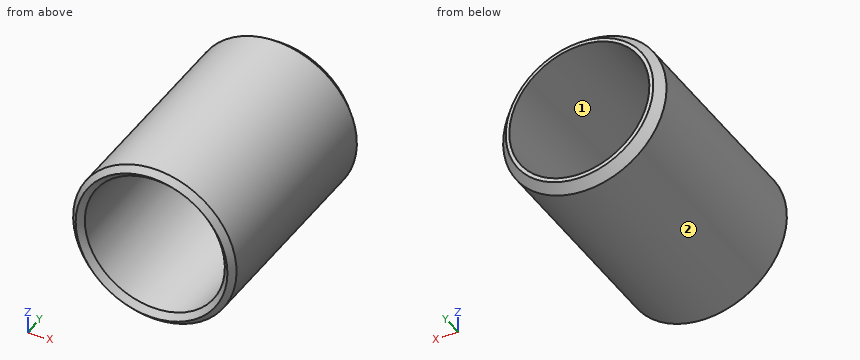
```python
from build123d import *

# Parameters (mm, degrees)
CROQUIS2_R            = 6
CORTAR_EXTRUIR1_DEPTH = 60
CHAFL_N2_SIZE         = 0.5
CHAFL_N2_SIZE_2       = 0.354903907


with BuildPart() as part:
    # Croquis1 → Revolución1 (revolve)
    with BuildSketch(Plane.XY, mode=Mode.PRIVATE) as revoluci_n1_sk:
        Polygon((-7, 18.808246407), (-7, 0), (0, 0), (0, 20), (-6, 20), align=None)
    revolve(revoluci_n1_sk.sketch.rotate(Axis((0, 0, 0), (0, 1, 0)), 270), axis=Axis((0, 0, 0), (0, 1, 0)))

    # Croquis2 → Cortar-Extruir1 (cut)
    with BuildSketch(Plane(origin=(0, 20, 0), x_dir=(1, 0, 0), z_dir=(0, 1, 0))):
        with Locations(Location((0, 0, 0), (0, 0, 270))):
            Circle(CROQUIS2_R)
    extrude(amount=-CORTAR_EXTRUIR1_DEPTH, mode=Mode.SUBTRACT)

    # Chaflán2
    # the kernel refuses this chamfer: 0.5, 0.354903907 mm, written as the material it takes off along each edge
    with BuildSketch(Plane(origin=(0, 0, 0), x_dir=(0, 0, 1), z_dir=(-1, 0, 0))) as chafl_n2_piece_1:
        Polygon((6 + CHAFL_N2_SIZE, 0), (6, CHAFL_N2_SIZE), (6, 0), align=None)
    revolve(axis=Axis((0, 0, 0), (0, 1, 0)), mode=Mode.SUBTRACT)
    with BuildSketch(Plane(origin=(0, 0, 0), x_dir=(0, 0, -1), z_dir=(1, 0, 0))) as chafl_n2_piece_2:
        Polygon((7, CHAFL_N2_SIZE), (7 - CHAFL_N2_SIZE, 0), (7, 0), align=None)
    revolve(axis=Axis((0, 0, 0), (0, 1, 0)), mode=Mode.SUBTRACT)
    with BuildSketch(Plane(origin=(0, 20, 0), x_dir=(0, 0, 1), z_dir=(-1, 0, 0))) as chafl_n2_piece_3:
        Polygon((6 + CHAFL_N2_SIZE * 0.642787609687, -CHAFL_N2_SIZE * 0.766044443119), (6, -CHAFL_N2_SIZE_2), (6, 0), align=None)
    revolve(axis=Axis((0, 20, 0), (0, 1, 0)), revolution_arc=180, mode=Mode.SUBTRACT)
    with BuildSketch(Plane(origin=(0, 20, 0), x_dir=(0, 0, -1), z_dir=(1, 0, 0))) as chafl_n2_piece_4:
        Polygon((6 + CHAFL_N2_SIZE * 0.642787609687, -CHAFL_N2_SIZE * 0.766044443119), (6, -CHAFL_N2_SIZE_2), (6, 0), align=None)
    revolve(axis=Axis((0, 20, 0), (0, 1, 0)), revolution_arc=180, mode=Mode.SUBTRACT)


solid = part.part
```
The model under review builds one solid part; all positions refer to its coordinate system, in mm. Face numbers are marked on the shaded views. Give positions to 0.01 mm unless a question says otherwise; leave off trailing zeros. Loops run counter-clockwise (first coordinate to the right, second up) from the corner with the lowest first, then second, coordinate; pieces in that order, holes last. Notation, with made-up numbers: (1.25, 63.25) -> (12.25, 63.25) arc R12 cw to (12.25, 77.25) -> close; hole circle Ø2 at (51.5, 35). An arc over 180 degrees is marked (long way). Use CSV: the item, a comma, the result in double quotes.
1. For P1, Ø3, axis at y = 14, z = -3, coming from the +X side; P2, Ø4, axis at x = 2, z = -2, coming from the +Y side; P3, Ø8, axis at x = 5.5, y = 13.5, coming from the -Z side, all flat-tipped, find the tip position at first contact; note any pin that passes through.
Result:
P1,"stops at x = 6.84"
P2,"passes through"
P3,"stops at z = -6.84"
2. To check wall thickness, follow probe 1 along X at (y, z) = (1.75, -0.25); probe 2 along Z at (x, y) = (0, 7.25); probe 3 along Z at (x, y) = (3, 4). State the ranges of each line that lie inside material, in increasing order. Write a range as from..to.
Result:
probe 1,"x = -7..-5.99, 5.99..7"
probe 2,"z = -7..-6, 6..7"
probe 3,"z = -6.32..-5.2, 5.2..6.32"
3. Consider section C-C, the plane y = 7.25. Write out the cut boundary in (x, z).
Result:
outline,"circle Ø14 at (0, 0); hole circle Ø12 at (0, 0)"
4. The part is to be moulded in two halves that separate along X. For the marked faces 1 and 2, say which applies: +X half, -X half, draft (parallel to the pull), parting line (faces both ways), or undercut.
Result:
face 1,"undercut"
face 2,"parting line"
5. Consider section B-B, the plane x = 0. Write out the cut boundary in (y, z).
Result:
outline,"(0, -6.5) -> (0.5, -7) -> (18.81, -7) -> (19.62, -6.32) -> (19.65, -6) -> (0.5, -6) -> close; (0, 6.5) -> (0.5, 6) -> (19.65, 6) -> (19.62, 6.32) -> (18.81, 7) -> (0.5, 7) -> close"
6. Consider section A-A, the plane z = 0. Write out the cut boundary in (x, y), then the cut area to 3 significant figures.
Result:
outline,"(-7, 0.5) -> (-6.5, 0) -> (-6, 0.5) -> (-6, 19.65) -> (-6.32, 19.62) -> (-7, 18.81) -> close; (6, 0.5) -> (6.5, 0) -> (7, 0.5) -> (7, 18.81) -> (6.32, 19.62) -> (6, 19.65) -> close"
area,"38.2 mm²"
